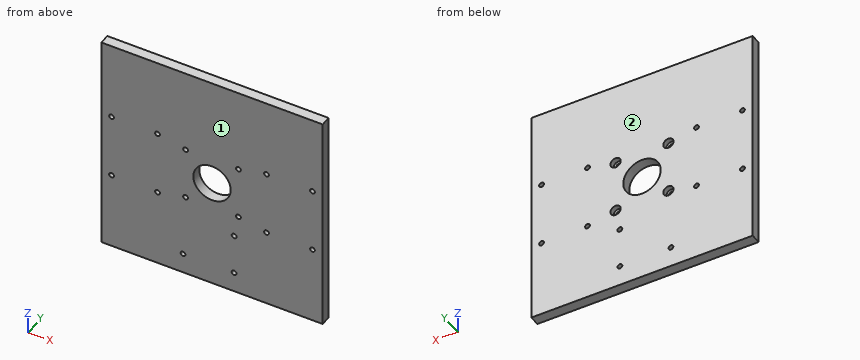
from build123d import *

# Parameters (mm, degrees)
SKETCH1_W           = 130
SKETCH1_H           = 130
SKETCH1_R           = 11
BOSS_EXTRUDE1_DEPTH = 6
SKETCH2_R           = 1.42
CUT_EXTRUDE1_DEPTH  = 6
SKETCH3_R           = 3
CUT_EXTRUDE2_DEPTH  = 3
SKETCH4_R           = 1.42
CUT_EXTRUDE3_DEPTH  = 10
SKETCH5_R           = 1.42
CUT_EXTRUDE4_DEPTH  = 10


with BuildPart() as part:
    # Sketch1 → Boss-Extrude1 (new body)
    with BuildSketch(Plane(origin=(0, 0, 0), x_dir=(1, 0, 0), z_dir=(0, 1, 0))):
        Rectangle(SKETCH1_W, SKETCH1_H)
        with Locations(Location((0, 0, 0), (0, 0, 270))):
            Circle(SKETCH1_R, mode=Mode.SUBTRACT)
    extrude(amount=BOSS_EXTRUDE1_DEPTH)

    # Sketch2 → Cut-Extrude1 (cut)
    with BuildSketch(Plane(origin=(0, 6, 0), x_dir=(1, 0, 0), z_dir=(0, 1, 0))):
        with Locations(Location((-15.5, 15.5, 0), (0, 0, 270))):
            Circle(SKETCH2_R)
        with Locations(Location((15.5, 15.5, 0), (0, 0, 270))):
            Circle(SKETCH2_R)
        with Locations(Location((15.5, -15.5, 0), (0, 0, 270))):
            Circle(SKETCH2_R)
        with Locations(Location((-15.5, -15.5, 0), (0, 0, 270))):
            Circle(SKETCH2_R)
    extrude(amount=-CUT_EXTRUDE1_DEPTH, mode=Mode.SUBTRACT)

    # Sketch3 → Cut-Extrude2 (cut)
    with BuildSketch(Plane(origin=(0, 6, 0), x_dir=(1, 0, 0), z_dir=(0, 1, 0))):
        with Locations(Location((-15.5, 15.5, 0), (0, 0, 270))):
            Circle(SKETCH3_R)
        with Locations(Location((15.5, 15.5, 0), (0, 0, 270))):
            Circle(SKETCH3_R)
        with Locations(Location((15.5, -15.5, 0), (0, 0, 270))):
            Circle(SKETCH3_R)
        with Locations(Location((-15.5, -15.5, 0), (0, 0, 270))):
            Circle(SKETCH3_R)
    extrude(amount=-CUT_EXTRUDE2_DEPTH, mode=Mode.SUBTRACT)

    # Sketch4 → Cut-Extrude3 (cut)
    with BuildSketch(Plane(origin=(0, 6, 0), x_dir=(1, 0, 0), z_dir=(0, 1, 0))):
        with Locations(Location((-59, 19, 0), (0, 0, 270))):
            Circle(SKETCH4_R)
        with Locations(Location((-32, 19, 0), (0, 0, 270))):
            Circle(SKETCH4_R)
        with Locations(Location((-32, -19, 0), (0, 0, 270))):
            Circle(SKETCH4_R)
        with Locations(Location((-59, -19, 0), (0, 0, 270))):
            Circle(SKETCH4_R)
        with Locations(Location((59, 19, 0), (0, 0, 90))):
            Circle(SKETCH4_R)
        with Locations(Location((59, -19, 0), (0, 0, 90))):
            Circle(SKETCH4_R)
        with Locations(Location((32, -19, 0), (0, 0, 90))):
            Circle(SKETCH4_R)
        with Locations(Location((32, 19, 0), (0, 0, 90))):
            Circle(SKETCH4_R)
    extrude(amount=-CUT_EXTRUDE3_DEPTH, mode=Mode.SUBTRACT)

    # Sketch5 → Cut-Extrude4 (cut)
    with BuildSketch(Plane(origin=(0, 6, 0), x_dir=(1, 0, 0), z_dir=(0, 1, 0))):
        with Locations(Location((13, 53, 0), (0, 0, 270))):
            Circle(SKETCH5_R)
        with Locations(Location((-17, 53, 0), (0, 0, 270))):
            Circle(SKETCH5_R)
        with Locations(Location((13, 29, 0), (0, 0, 270))):
            Circle(SKETCH5_R)
    extrude(amount=-CUT_EXTRUDE4_DEPTH, mode=Mode.SUBTRACT)


solid = part.part
The model under review builds one solid part; all positions refer to its coordinate system, in mm. Face numbers are marked on the shaded views. Coordinates: 2 decimals unless noted, no trailing zeros. Order: outer loops, then holes, each group sorted by start corner. A loop starts at its lowest first (then second) coordinate and runs counter-clockwise, first axis right, second up. Notation, with made-up numbers: (-35.5, -13.5) -> (-19.5, -13.5) arc R26 ccw to (-19.5, 2.5) -> close; hole circle Ø5 at (15.25, -31.5). An arc over 180 degrees is marked (long way). Answer in a Markdown table with one row per item.
(1) Consider section B-B (z = 0). Write out the cut boundary in (x, y).
Answers:
| item | result |
|---|---|
| outline | (-65, 0) -> (-11, 0) -> (-11, 6) -> (-65, 6) -> close; (11, 0) -> (65, 0) -> (65, 6) -> (11, 6) -> close |
(2) Wall thickness on line 1 along X through (y, z) = (1.2, -19); line 2 along X through (y, z) = (1.1, 15.5); line 3 along Z through (x, y) = (12, 1.15): over which ranges is each line inside the solid? List them lowest first.
Answers:
| item | result |
|---|---|
| line 1 | -65 to -60.42, -57.58 to -33.42, -30.58 to 30.58, 33.42 to 57.58, 60.42 to 65 |
| line 2 | -65 to -16.92, -14.08 to 14.08, 16.92 to 65 |
| line 3 | -65 to -54.01, -51.99 to -30.01, -27.99 to 65 |
(3) Insertion check: pin 1 (2.5 mm diameter, centred on x = -32, z = -19, fed in from +Y); pin 2 (1.5 mm diameter, centred on x = 32.5, z = 41.5, fed in from -Y). Each pin has a flat end and moves straight along its axis. Give the tip position at first contact, or say it passes through.
Answers:
| item | result |
|---|---|
| pin 1 | through |
| pin 2 | y = 0 |
(4) The part is to be moulded in two halves that separate along Y. For the marked faces 1 and 2, say which applies: +Y half, -Y half, draft (parallel to the pull), parting line (faces both ways), or undercut.
Answers:
| item | result |
|---|---|
| face 1 | -Y half |
| face 2 | +Y half |
(5) Consider section C-C (y = 1.2). State how many separate pieces and enclosed holes the cut face has, plus the area to 3 significant figures.
Answers:
| item | result |
|---|---|
| separate pieces | 1 |
| enclosed holes | 16 |
| area | 16,400 mm² |
(6) Consider section A-A (x = 0). Write out the cut boundary in (y, z).
Answers:
| item | result |
|---|---|
| outline | (0, -65) -> (6, -65) -> (6, -11) -> (0, -11) -> close; (0, 11) -> (6, 11) -> (6, 65) -> (0, 65) -> close |
